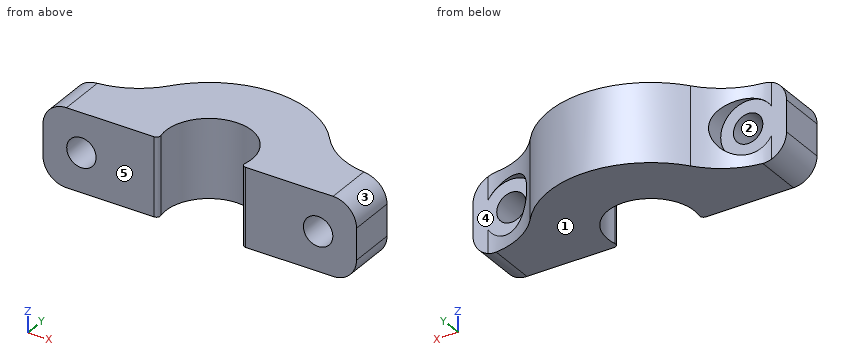
```python
from build123d import *

# Parameters (mm, degrees)
BOSS_EXTRUDE1_START      = -1
SKETCH1_W                = 40
SKETCH1_H                = 10
BOSS_EXTRUDE1_DEPTH      = 5
BOSS_EXTRUDE2_DEPTH      = 5
BOSS_EXTRUDE2_DEPTH_BACK = 5
SKETCH3_W                = 10
SKETCH3_H                = 10
BOSS_EXTRUDE3_DEPTH      = 7
FILLET1_R                = 3
FILLET2_R                = 3
FILLET4_R                = 10
CUT_EXTRUDE1_DEPTH       = 26.973833083
CUT_EXTRUDE1_DEPTH_BACK  = 26.973833083
SKETCH4_R                = 1.875
CUT_EXTRUDE2_START       = 7
SKETCH5_R                = 3.5
CUT_EXTRUDE2_DEPTH       = 10
SKETCH9_W                = 47.094451366
SKETCH9_H                = 23.336565295
CUT_EXTRUDE5_DEPTH       = 1
FILLET5_R                = 0.5
SKETCH7_W                = 51.703075982
SKETCH7_H                = 23.04476915
CUT_EXTRUDE4_DEPTH       = 26.973833083


with BuildPart() as part:
    # Sketch1 → Boss-Extrude1 (new body)
    with BuildSketch(Plane(origin=(0, 0, 0), x_dir=(1, 0, 0), z_dir=(0, 1, 0)).offset(BOSS_EXTRUDE1_START)):
        Rectangle(SKETCH1_W, SKETCH1_H)
    extrude(amount=-BOSS_EXTRUDE1_DEPTH)

    # Fillet2
    fillet2_edges = [part.edges().sort_by_distance(p)[0] for p in [
        (20, -3.5, 5),
        (-20, -3.5, 5),
        (-20, -3.5, -5),
        (20, -3.5, -5),
    ]]
    fillet(fillet2_edges, radius=FILLET2_R)


with BuildPart() as body_2:
    # Sketch2 → Boss-Extrude2 (new, two sides: drawn at the far end of the back side and taken through both)
    with BuildSketch(Plane.XY.offset(-BOSS_EXTRUDE2_DEPTH_BACK)):
        with BuildLine():
            Line((-12.694880858, 0), (-4.733920151, 0))
            ThreePointArc((-4.733920151, 0), (0, 8.3), (4.733920151, 0))
            Line((4.733920151, 0), (12.694880858, 0))
            ThreePointArc((12.694880858, 0), (0, 15.8), (-12.694880858, 0))
        make_face()
    extrude(amount=BOSS_EXTRUDE2_DEPTH + BOSS_EXTRUDE2_DEPTH_BACK)

    # Sketch3 → Boss-Extrude3 (add)
    with BuildSketch(Plane(origin=(0, 0, 0), x_dir=(1, 0, 0), z_dir=(0, 1, 0))):
        with Locations((-15, 0)):
            Rectangle(SKETCH3_W, SKETCH3_H)
        with Locations((15, 0)):
            Rectangle(SKETCH3_W, SKETCH3_H)
    extrude(amount=BOSS_EXTRUDE3_DEPTH)

    # Fillet1
    fillet1_edges = [body_2.edges().sort_by_distance(p)[0] for p in [
        (-20, 3.5, -5),
        (-20, 3.5, 5),
        (20, 3.5, 5),
        (20, 3.5, -5),
    ]]
    fillet(fillet1_edges, radius=FILLET1_R)

    # Fillet4
    fillet4_edges = [body_2.edges().sort_by_distance(p)[0] for p in [
        (12.302845199, 7, 0),
        (-12.302845199, 7, 0),
    ]]
    fillet(fillet4_edges, radius=FILLET4_R)


with BuildPart() as cut_extrude1_tool:
    # Sketch4 → Cut-Extrude1 (new, two sides: drawn at the far end of the back side and taken through both)
    with BuildSketch(Plane(origin=(0, 0, 0), x_dir=(1, 0, 0), z_dir=(0, 1, 0)).offset(-CUT_EXTRUDE1_DEPTH_BACK)):
        with Locations(Location((-15.1, 0, 0), (0, 0, 270))):
            Circle(SKETCH4_R)
        with Locations(Location((15.1, 0, 0), (0, 0, 270))):
            Circle(SKETCH4_R)
    extrude(amount=CUT_EXTRUDE1_DEPTH + CUT_EXTRUDE1_DEPTH_BACK)


with BuildPart() as part_1:
    add(part.part)

    # Cut-Extrude1: cut by cut_extrude1_tool
    add(cut_extrude1_tool.part, mode=Mode.SUBTRACT)

    # Sketch7 → Cut-Extrude4 (cut, through all)
    with BuildSketch(Plane(origin=(0, 0, 0), x_dir=(1, 0, 0), z_dir=(0, 1, 0))):
        with Locations((-1.693322056, -1.721439234)):
            Rectangle(SKETCH7_W, SKETCH7_H)
    extrude(amount=-CUT_EXTRUDE4_DEPTH, mode=Mode.SUBTRACT)


with BuildPart() as body_2_1:
    add(body_2.part)

    # Cut-Extrude1: cut by cut_extrude1_tool
    add(cut_extrude1_tool.part, mode=Mode.SUBTRACT)

    # Sketch5 → Cut-Extrude2 (cut)
    with BuildSketch(Plane(origin=(0, 0, 0), x_dir=(1, 0, 0), z_dir=(0, 1, 0)).offset(CUT_EXTRUDE2_START)):
        with Locations((-15.1, 0)):
            Circle(SKETCH5_R)
        with Locations((15.1, 0)):
            Circle(SKETCH5_R)
    extrude(amount=CUT_EXTRUDE2_DEPTH, mode=Mode.SUBTRACT)

    # Sketch9 → Cut-Extrude5 (cut)
    with BuildSketch(Plane(origin=(0, 0, 0), x_dir=(1, 0, 0), z_dir=(0, 1, 0))):
        with Locations((2.081495267, 0.004136026)):
            Rectangle(SKETCH9_W, SKETCH9_H)
    extrude(amount=CUT_EXTRUDE5_DEPTH, mode=Mode.SUBTRACT)

    # Fillet5
    fillet5_edges = [body_2_1.edges().sort_by_distance(p)[0] for p in [
        (-5.197114584, 1, 0),
        (5.197114584, 1, 0),
    ]]
    fillet(fillet5_edges, radius=FILLET5_R)


solid = body_2_1.part
```
The listing builds one solid part. Answer for the finished solid, in the listing's coordinates (mm). Face numbers are marked on the shaded views. A direction names the side the tool comes from. Round coordinates to 2 decimals unless told otherwise and drop trailing zeros. Loops run counter-clockwise (first coordinate to the right, second up) from the corner with the lowest first, then second, coordinate; pieces in that order, holes last.
Q1. Section C-C, the plane x = -16 is taken. Determine the outline of the cut face in (y, z), then the cut area to 3 significant figures.
Q2. Find the intervals of material crossed by line 1 (X direction, y = 3, z = 0) (3 decimals); line 2 (Z direction, x = -15.1, y = 3.5) (3 decimals); line 3 (X direction, y = 3.5, z = 0.5), in increasing order.
Q3. Section D-D, the plane y = 5.5 is taken. Determine the outline of the cut face in (x, z) (3 decimals), then the cut area to 3 significant figures.
Q4. Section A-A, the plane y = 2.8 is taken. Determine the outline of the cut face in (x, z) (3 decimals).
Q5. Section B-B, the plane z = -0.25 is taken. Determine the outline of the cut face in (x, y), then the cut area to 3 significant figures.
Q6. Which of the six approach directions +Z, -Z, +X, -X, +Y, -Y give full straight-line access (tool end or side, diameter ignored) to the marked faces 4 and 5?
Q7. For a pull along Z with two mould halves and no side action, classify the marked faces 1, 2 and 3 as released by +Z, released by -Z, zero draft, split by the parting line, or undercut.
Q8. Given pin 1 Ø2.5 at (x, z) = (17, 0.5) entering from +Y; pin 2 Ø3 at (x, z) = (-4, 2.5) entering from +Y, each flat-ended and moving along its own axis, determine where each tip first touches the part or whether it passes through.
Completed:
1. outline: (1, -5) - (7.22, -5) - (7.22, -3.38) - (7, -3.38) - (7, -1.64) - (1, -1.64) - close; (1, 1.64) - (7, 1.64) - (7, 3.38) - (7.22, 3.38) - (7.22, 5) - (1, 5) - close
1. area: 41.0 mm2
2. line 1: x = -20 to -16.975, -13.225 to -5.496, 5.496 to 13.225, 16.975 to 20
2. line 2: z = -5 to -1.875, 1.875 to 5
2. line 3: x = -20 to -16.91, -13.29 to -5.46, 5.46 to 13.29, 16.91 to 20
3. outline: (-20, -2) arc R3 ccw to (-17, -5) - (-4.792, -5) - (-4.792, 5) - (-17, 5) arc R3 ccw to (-20, 2) - close; (4.792, -5) - (17, -5) arc R3 ccw to (20, -2) - (20, 2) arc R3 ccw to (17, 5) - (4.792, 5) - close; hole circle Ø3.75 at (-15.1, 0); hole circle Ø3.75 at (15.1, 0)
3. area: 274 mm2
4. outline: (-20, -2) arc R3 ccw to (-17, -5) - (-5.5, -5) - (-5.5, 5) - (-17, 5) arc R3 ccw to (-20, 2) - close; (5.5, -5) - (17, -5) arc R3 ccw to (20, -2) - (20, 2) arc R3 ccw to (17, 5) - (5.5, 5) - close; hole circle Ø3.75 at (-15.1, 0); hole circle Ø3.75 at (15.1, 0)
5. outline: (-20, 1) - (-16.96, 1) - (-16.96, 7) - (-20, 7) - close; (-13.24, 1) - (-5.86, 1) arc R0.5 ccw to (-5.37, 1.61) arc R5.5 cw (long way) to (5.37, 1.61) arc R0.5 ccw to (5.86, 1) - (13.24, 1) - (13.24, 7) - (11.61, 7) - (11.61, 9.39) arc R10 cw to (10.23, 10.83) arc R13 ccw to (-10.23, 10.83) arc R10 cw to (-11.61, 9.39) - (-11.61, 7) - (-13.24, 7) - close; (16.96, 1) - (20, 1) - (20, 7) - (16.96, 7) - close
5. area: 286 mm2
6. face 4: +Y
6. face 5: +Z, -Z, +X, -X, -Y
7. face 1: released by -Z
7. face 2: undercut
7. face 3: released by +Z
8. pin 1: stops at y = 7
8. pin 2: stops at y = 15.56
